```python
from build123d import *

# Parameters (mm, degrees)
SKETCH1_W           = 190.5
SKETCH1_H           = 190.5
BOSS_EXTRUDE1_DEPTH = 9.525
SKETCH2_W           = 9.525
SKETCH2_H           = 38.1
CUT_EXTRUDE1_DEPTH  = 9.525
SKETCH3_W           = 9.525
SKETCH3_H           = 38.1
CUT_EXTRUDE2_DEPTH  = 9.525
SKETCH4_W           = 9.525
SKETCH4_H           = 38.1
CUT_EXTRUDE3_DEPTH  = 9.525
SKETCH5_W           = 9.525
SKETCH5_H           = 38.1
CUT_EXTRUDE4_DEPTH  = 9.525
SKETCH6_W           = 9.525
SKETCH6_H           = 38.1
CUT_EXTRUDE5_DEPTH  = 9.525
SKETCH7_W           = 9.525
SKETCH7_H           = 38.1
CUT_EXTRUDE6_DEPTH  = 9.525
SKETCH8_W           = 28.575
SKETCH8_H           = 9.525
CUT_EXTRUDE7_DEPTH  = 9.525
SKETCH9_W           = 38.1
SKETCH9_H           = 9.525
CUT_EXTRUDE8_DEPTH  = 9.525
SKETCH10_W          = 28.575
SKETCH10_H          = 9.525
CUT_EXTRUDE9_DEPTH  = 9.525
SKETCH11_W          = 28.575
SKETCH11_H          = 9.525
CUT_EXTRUDE11_DEPTH = 9.525
SKETCH12_W          = 38.1
SKETCH12_H          = 9.525
CUT_EXTRUDE12_DEPTH = 9.525
SKETCH14_W          = 28.575
SKETCH14_H          = 9.525
CUT_EXTRUDE13_DEPTH = 9.525
SKETCH15_W          = 68.2625
SKETCH15_H          = 23.8125
CUT_EXTRUDE14_DEPTH = 9.525
SKETCH16_W          = 82.55
SKETCH16_H          = 31.75
CUT_EXTRUDE15_DEPTH = 9.525


with BuildPart() as part:
    # Sketch1 → Boss-Extrude1 (new body)
    with BuildSketch(Plane(origin=(0, 0, 0), x_dir=(1, 0, 0), z_dir=(0, 1, 0))):
        with Locations((-91.022160665, 92.07132964)):
            Rectangle(SKETCH1_W, SKETCH1_H)
    extrude(amount=BOSS_EXTRUDE1_DEPTH)

    # Sketch2 → Cut-Extrude1 (cut)
    with BuildSketch(Plane(origin=(0, 9.525, 0), x_dir=(1, 0, 0), z_dir=(0, 1, 0))):
        with Locations((-0.534660665, 15.87132964)):
            Rectangle(SKETCH2_W, SKETCH2_H)
    extrude(amount=-CUT_EXTRUDE1_DEPTH, mode=Mode.SUBTRACT)

    # Sketch3 → Cut-Extrude2 (cut)
    with BuildSketch(Plane(origin=(0, 9.525, 0), x_dir=(1, 0, 0), z_dir=(0, 1, 0))):
        with Locations((-0.534660665, 92.07132964)):
            Rectangle(SKETCH3_W, SKETCH3_H)
    extrude(amount=-CUT_EXTRUDE2_DEPTH, mode=Mode.SUBTRACT)

    # Sketch4 → Cut-Extrude3 (cut)
    with BuildSketch(Plane(origin=(0, 9.525, 0), x_dir=(1, 0, 0), z_dir=(0, 1, 0))):
        with Locations((-0.534660665, 168.27132964)):
            Rectangle(SKETCH4_W, SKETCH4_H)
    extrude(amount=-CUT_EXTRUDE3_DEPTH, mode=Mode.SUBTRACT)

    # Sketch5 → Cut-Extrude4 (cut)
    with BuildSketch(Plane.XZ):
        with Locations((-181.509660665, -15.87132964)):
            Rectangle(SKETCH5_W, SKETCH5_H)
    extrude(amount=-CUT_EXTRUDE4_DEPTH, mode=Mode.SUBTRACT)

    # Sketch6 → Cut-Extrude5 (cut)
    with BuildSketch(Plane.XZ):
        with Locations((-181.509660665, -92.07132964)):
            Rectangle(SKETCH6_W, SKETCH6_H)
    extrude(amount=-CUT_EXTRUDE5_DEPTH, mode=Mode.SUBTRACT)

    # Sketch7 → Cut-Extrude6 (cut)
    with BuildSketch(Plane.XZ):
        with Locations((-181.509660665, -168.27132964)):
            Rectangle(SKETCH7_W, SKETCH7_H)
    extrude(amount=-CUT_EXTRUDE6_DEPTH, mode=Mode.SUBTRACT)

    # Sketch8 → Cut-Extrude7 (cut)
    with BuildSketch(Plane.XZ):
        with Locations((-19.584660665, -182.55882964)):
            Rectangle(SKETCH8_W, SKETCH8_H)
    extrude(amount=-CUT_EXTRUDE7_DEPTH, mode=Mode.SUBTRACT)

    # Sketch9 → Cut-Extrude8 (cut)
    with BuildSketch(Plane.XZ):
        with Locations((-91.022160665, -182.55882964)):
            Rectangle(SKETCH9_W, SKETCH9_H)
    extrude(amount=-CUT_EXTRUDE8_DEPTH, mode=Mode.SUBTRACT)

    # Sketch10 → Cut-Extrude9 (cut)
    with BuildSketch(Plane.XZ):
        with Locations((-162.459660665, -182.55882964)):
            Rectangle(SKETCH10_W, SKETCH10_H)
    extrude(amount=-CUT_EXTRUDE9_DEPTH, mode=Mode.SUBTRACT)

    # Sketch11 → Cut-Extrude11 (cut)
    with BuildSketch(Plane(origin=(0, 0, 0), x_dir=(-1, 0, 0), z_dir=(0, -1, 0))):
        with Locations((162.459660665, 1.58382964)):
            Rectangle(SKETCH11_W, SKETCH11_H)
    extrude(amount=-CUT_EXTRUDE11_DEPTH, mode=Mode.SUBTRACT)

    # Sketch12 → Cut-Extrude12 (cut)
    with BuildSketch(Plane.XZ):
        with Locations((-91.022160665, -1.58382964)):
            Rectangle(SKETCH12_W, SKETCH12_H)
    extrude(amount=-CUT_EXTRUDE12_DEPTH, mode=Mode.SUBTRACT)

    # Sketch14 → Cut-Extrude13 (cut)
    with BuildSketch(Plane(origin=(0, 0, 0), x_dir=(-1, 0, 0), z_dir=(0, -1, 0))):
        with Locations((19.584660665, 1.58382964)):
            Rectangle(SKETCH14_W, SKETCH14_H)
    extrude(amount=-CUT_EXTRUDE13_DEPTH, mode=Mode.SUBTRACT)

    # Sketch15 → Cut-Extrude14 (cut)
    with BuildSketch(Plane.XZ):
        with Locations((-90.276924716, -130.287204322)):
            Rectangle(SKETCH15_W, SKETCH15_H)
    extrude(amount=-CUT_EXTRUDE14_DEPTH, mode=Mode.SUBTRACT)

    # Sketch16 → Cut-Extrude15 (cut)
    with BuildSketch(Plane.XZ):
        with Locations((-91.083368355, -83.846953715)):
            Rectangle(SKETCH16_W, SKETCH16_H)
    extrude(amount=-CUT_EXTRUDE15_DEPTH, mode=Mode.SUBTRACT)


solid = part.part
```
Design review of the part built by this model. Coordinates are the model's own, in mm. A direction names the side the tool comes from. Give positions to 0.01 mm unless a question says otherwise; leave off trailing zeros. Order: outer loops, then holes, each group sorted by start corner. A loop starts at its lowest first (then second) coordinate and runs counter-clockwise, first axis right, second up. Notation, with made-up numbers: (72.5, 7.5) -> (96.5, 7.5) arc R17 ccw to (96.5, 11.5) -> close; hole circle Ø11 at (4.25, 14). An arc over 180 degrees is marked (long way). Write item = value, one per line. Start each with the question number.
(1) We need section B-B on z = -123.5. Write out the cut boundary in (x, y) (3 decimals).
(2) We need section C-C on x = -75. Write out the cut boundary in (y, z) (3 decimals).
(3) For faces 1 (the face through (-124.408, 5, -130)), 2 (the face through (-162, 5, -6.346)), 3 (the face through (-71.972, 5, -183)), 4 (the face through (-19, 5, -6.346)), 5 (the face through (-71.972, 5, -2)), list the 3-axis set-ups (+Z, -Z, +X, -X, +Y, -Y) from which the entire face can be reached by the end or side of a thin tool; tool diameter is ignored.
(4) We need section D-D on y = 2.5. State how many separate pieces and enclosed holes the cut face has, plus the area to 3 significant figures.
(5) To check wall thickness, follow line 1 along Z through (x, y) = (-84, 2); line 2 along Z through (x, y) = (-67, 6.25); line 3 along X through (y, z) = (0.5, -96). State the ranges of each line that lie inside material, in increasing order.
(6) For pin 1 (5 mm diameter, centred on y = 5, z = -1.5, fed in from +X); pin 2 (3 mm diameter, centred on x = -98, y = 1.5, fed in from -Z); pin 3 (5 mm diameter, centred on x = -1.5, y = 6, fed in from -Z), all flat-tipped, find the tip position at first contact; note any pin that passes through.
(7) Mouldability with a two-part tool opening along X and no side actions: class faces 6 (the face through (-5.297, 5, -163)), 7 (the face through (-20, 5, -177.796)), 8 (the face through (-110.072, 5, -2)), 9 (the face through (-91, 5, -142.193)) as +X half, -X half, draft (parallel to the pull), parting line (faces both ways), or undercut.
(8) We need section A-A on x = -127. Write out the cut boundary in (y, z) (3 decimals).
Numbers:
q1.outline = (-186.272, 0) -> (-124.408, 0) -> (-124.408, 9.525) -> (-186.272, 9.525) -> close; (-56.146, 0) -> (4.228, 0) -> (4.228, 9.525) -> (-56.146, 9.525) -> close
q2.outline = (0, -177.796) -> (9.525, -177.796) -> (9.525, -142.193) -> (0, -142.193) -> close; (0, -118.381) -> (9.525, -118.381) -> (9.525, -99.722) -> (0, -99.722) -> close; (0, -67.972) -> (9.525, -67.972) -> (9.525, -6.346) -> (0, -6.346) -> close
q3.face_1 = +Y, -Y
q3.face_2 = +Z, -X, +Y, -Y
q3.face_3 = -Z, +Y, -Y
q3.face_4 = +Z, +X, +Y, -Y
q3.face_5 = +Z, +Y, -Y
q4.separate_pieces = 1
q4.enclosed_holes = 2
q4.area = 28,100 mm^2
q5.line_1 = -177.8 to -142.19, -118.38 to -99.72, -67.97 to -6.35
q5.line_2 = -187.32 to -142.19, -118.38 to -99.72, -67.97 to 3.18
q5.line_3 = -176.75 to -132.36, -49.81 to -5.3
q6.pin_1 = -33.87
q6.pin_2 = -177.8
q6.pin_3 = -149.22
q7.face_6 = +X half
q7.face_7 = draft
q7.face_8 = undercut
q7.face_9 = undercut
q8.outline = (0, -187.321) -> (9.525, -187.321) -> (9.525, -99.722) -> (0, -99.722) -> close; (0, -67.972) -> (9.525, -67.972) -> (9.525, 3.179) -> (0, 3.179) -> close
